The listing builds one solid part. Answer for the finished solid, in the listing's coordinates (mm). A direction names the side the tool comes from. Give positions to 0.01 mm unless a question says otherwise; leave off trailing zeros. Order: outer loops, then holes, each group sorted by start corner. A loop starts at its lowest first (then second) coordinate and runs counter-clockwise, first axis right, second up.
```python
from build123d import *


with BuildPart() as part:
    # Sketch → Revolution (revolve)
    with BuildSketch(Plane.XZ):
        Polygon((0, 30), (5, 30), (5, 0), (10, 0), (30, 20), (25, 25), (8, 8), (8, 47.5), (17.5, 57), (12.5, 62), (5, 54.5), (5, 95), (0, 95), align=None)
    revolve(axis=Axis((0, 0, 0), (0, 0, 1)))


solid = part.part
```
1) Find section C-C (y = 0). Write down the section's boundary in (x, z).
Geometry says:
outline: (-30, 20) - (-10, 0) - (-5, 0) - (-5, 30) - (5, 30) - (5, 0) - (10, 0) - (30, 20) - (25, 25) - (8, 8) - (8, 47.5) - (17.5, 57) - (12.5, 62) - (5, 54.5) - (5, 95) - (-5, 95) - (-5, 54.5) - (-12.5, 62) - (-17.5, 57) - (-8, 47.5) - (-8, 8) - (-25, 25) - close
2) For a pull along X with two mould halves and no side action, classify faces 5 (the cylindrical face through (-1.08, -4.88, 14.79)), 6 (the flat face through (-2, 5, 0)), 7 (the conical face through (-10.11, -7.75, 61.76)) as +X half, -X half, draft (parallel to the pull), parting line (faces both ways), or undercut.
Geometry says:
face 5: undercut
face 6: draft
face 7: parting line
3) Find section B-B (z = 12.5). Write down the section's boundary in (x, y).
Geometry says:
outline: circle Ø45 at (0, 0); circle Ø16 at (0, 0); hole circle Ø25 at (0, 0); hole circle Ø10 at (0, 0)
4) Given P1, Ø8, axis at y = -2.5, z = 54.5, coming from the -X side; P2, Ø6, axis at x = 12, z = 24.5, coming from the -Y side; P3, Ø8, axis at y = 22.5, z = 15, coming from the +X side; P4, Ø13, axis at x = 0, y = 0, coming from the -Z side, each flat-ended and moving along its own axis, determine where each tip first touches the part or whether it passes through.
Geometry says:
P1: stops at x = -17.5
P2: stops at y = -26.11
P3: stops at x = 19.78
P4: stops at z = 0
5) A tool of negligible diameter and unlimited length cuts with its end or side. For faces 1 (the flat face through (0, 0, 30)), 2 (the cylindrical face through (-1.08, -4.88, 75.03)), 3 (the flat face through (0, 0, 95)), 4 (the conical face through (-1.863, -8.39, 48.094)), from which of +Z, -Z, +X, -X, +Y, -Y can it reach the whole face along a straight path? Write none if from no direction.
Geometry says:
face 1: -Z
face 2: +Z
face 3: +Z, +X, -X, +Y, -Y
face 4: none
6) Straight lines are drawn through the part: probe 1 along Y at (x, z) = (0, 7.5); probe 2 along Y at (x, z) = (0, 19.25); probe 3 along Y at (x, z) = (0, 17.25). For each, find the intervals that lie inside material, in ascending order.
Geometry says:
probe 1: y = -17.5 to -5, 5 to 17.5
probe 2: y = -29.25 to -19.25, -8 to -5, 5 to 8, 19.25 to 29.25
probe 3: y = -27.25 to -17.25, -8 to -5, 5 to 8, 17.25 to 27.25
7) Find section A-A (z = 60). Write down the section's boundary in (x, y).
Geometry says:
outline: circle Ø29 at (0, 0); circle Ø10 at (0, 0); hole circle Ø21 at (0, 0)
